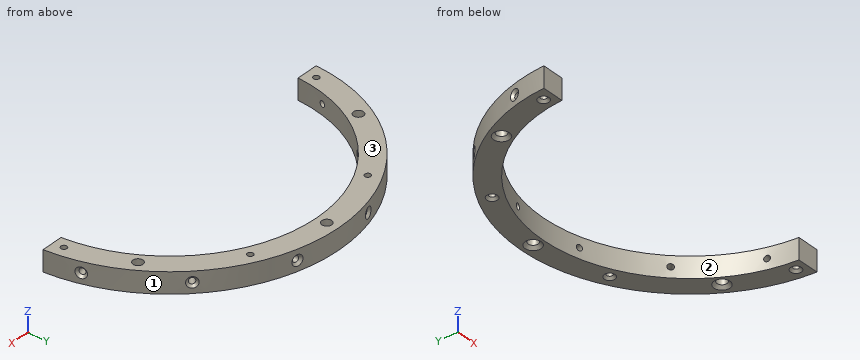
from build123d import *

# Parameters (mm, degrees)
BOSS_EXTRUDE1_DEPTH              = 3.96875
CIRPATTERN1_COUNT                = 6
CIRPATTERN1_ANGLE                = 150
F_4_40_TAPPED_HOLE3_D            = 2.2606
F_4_40_TAPPED_HOLE3_CSINK_D      = 4.1148
F_4_40_TAPPED_HOLE3_CSINK_ANGLE  = 90
CIRPATTERN2_COUNT                = 4
CIRPATTERN2_ANGLE                = 165
F_10_24_TAPPED_HOLE1_D           = 3.7973
F_10_24_TAPPED_HOLE1_CSINK_D     = 6.096
F_10_24_TAPPED_HOLE1_CSINK_ANGLE = 90
CIRPATTERN3_COUNT                = 3
CIRPATTERN3_ANGLE                = 120


with BuildPart() as part:
    # Sketch1 → Boss-Extrude1 (new body, symmetric)
    with BuildSketch(Plane.XY):
        with BuildLine():
            Line((-64.387964714, 3.8), (-55.87092267, 3.8))
            ThreePointArc((-55.87092267, 3.8), (0, 56), (55.87092267, 3.8))
            Line((55.87092267, 3.8), (64.387964714, 3.8))
            ThreePointArc((64.387964714, 3.8), (0, 64.5), (-64.387964714, 3.8))
        make_face()
    extrude(amount=BOSS_EXTRUDE1_DEPTH, both=True)

    # Sketch3 → #4-40 Tapped Hole2 (revolve, cut)
    with BuildSketch(Plane(origin=(62.302215796, 16.693828409, 0), x_dir=(-0.258819045, 0.965925826, 0), z_dir=(0, 0, 1))):
        Polygon((0, 0), (0, 9.549152758), (1.1303, 8.87), (1.1303, 0.9271), (2.0574, 0), align=None)
    f_4_40_tapped_hole2 = revolve(axis=Axis((68.435844793, 18.337329346, 0), (-0.965925826, -0.258819045, 0)), mode=Mode.SUBTRACT)

    # CirPattern1: #4-40 Tapped Hole2 ×6 about axis
    cirpattern1_axis = Axis((0, 0, 3.96875), (0, 0, 1))
    for i in range(1, CIRPATTERN1_COUNT):
        add(f_4_40_tapped_hole2.rotate(cirpattern1_axis, i * CIRPATTERN1_ANGLE / (CIRPATTERN1_COUNT - 1)), mode=Mode.SUBTRACT)

    # #4-40 Tapped Hole3 (through all)
    with Locations(Plane(origin=(0, 0, -3.96875), x_dir=(-1, 0, 0), z_dir=(0, 0, -1))):
        with Locations((-59.486691682, 7.831571533)):
            f_4_40_tapped_hole3 = CounterSinkHole(F_4_40_TAPPED_HOLE3_D / 2, F_4_40_TAPPED_HOLE3_CSINK_D / 2, counter_sink_angle=F_4_40_TAPPED_HOLE3_CSINK_ANGLE)

    # CirPattern2: #4-40 Tapped Hole3 ×4 about axis
    cirpattern2_axis = Axis((0, 0, 0), (0, 0, 1))
    for i in range(1, CIRPATTERN2_COUNT):
        add(f_4_40_tapped_hole3.rotate(cirpattern2_axis, i * CIRPATTERN2_ANGLE / (CIRPATTERN2_COUNT - 1)), mode=Mode.SUBTRACT)

    # #10-24 Tapped Hole1 (through all)
    with Locations(Plane(origin=(0, 0, -3.96875), x_dir=(-1, 0, 0), z_dir=(0, 0, -1))):
        with Locations((-51.961524227, 30)):
            f_10_24_tapped_hole1 = CounterSinkHole(F_10_24_TAPPED_HOLE1_D / 2, F_10_24_TAPPED_HOLE1_CSINK_D / 2, counter_sink_angle=F_10_24_TAPPED_HOLE1_CSINK_ANGLE)

    # CirPattern3: #10-24 Tapped Hole1 ×3 about axis
    cirpattern3_axis = Axis((0, 0, 0), (0, 0, 1))
    for i in range(1, CIRPATTERN3_COUNT):
        add(f_10_24_tapped_hole1.rotate(cirpattern3_axis, i * CIRPATTERN3_ANGLE / (CIRPATTERN3_COUNT - 1)), mode=Mode.SUBTRACT)


solid = part.part
CAD build for the part. Positions are in the model's coordinates, mm. Face numbers are marked on the shaded views. Give positions to 0.01 mm unless a question says otherwise; leave off trailing zeros. Order: outer loops, then holes, each group sorted by start corner. A loop starts at its lowest first (then second) coordinate and runs counter-clockwise, first axis right, second up. Notation, with made-up numbers: (68, 47) -> (121, 47) arc R8 cw to (121, 51) -> close; hole circle Ø9 at (39, 11). An arc over 180 degrees is marked (long way). Return JSON: item names as keys, results as strings.
Q1. Drill centre lines: line 1 (X direction, y = 30, z = -1); line 2 (X direction, y = 31.5, z = -3); line 3 (Y direction, x = 56.5, z = 1). Where is each one in solid material? Low to high.
Working result:
{"line 1": "-57.1 to -53.86, -50.06 to -47.29, 47.29 to 50.06, 53.86 to 57.1", "line 2": "-56.28 to -53.4, -50.52 to -46.3, 46.3 to 50.52, 53.4 to 56.28", "line 3": "3.8 to 14.59, 15.68 to 31.11"}
Q2. Saw through at A-A (y = 20). Write the cut outline in (x, z), then the cut area to 3 significant figures.
Working result:
{"outline": "(-61.32, -3.97) -> (-52.31, -3.97) -> (-52.31, 3.97) -> (-61.32, 3.97) -> close; (52.31, -3.97) -> (61.32, -3.97) -> (61.32, 3.97) -> (52.31, 3.97) -> close", "area": "143 mm²"}
Q3. Mould opens along X. For the marked faces 1, 2 and 3 say: pulls with the +X half, pulls with the -X half, needs draft (parallel to the pull), parting line crosses it, or undercut.
Working result:
{"face 1": "parting line crosses it", "face 2": "undercut", "face 3": "needs draft"}
Q4. Saw through at B-B (y = 30). Write the cut outline in (x, z), then the cut area to 3 significant figures.
Working result:
{"outline": "(-57.1, -3.97) -> (-55.01, -3.97) -> (-53.86, -2.82) -> (-53.86, 3.97) -> (-57.1, 3.97) -> close; (-50.06, -2.82) -> (-48.91, -3.97) -> (-47.29, -3.97) -> (-47.29, 3.97) -> (-50.06, 3.97) -> close; (47.29, -3.97) -> (48.91, -3.97) -> (50.06, -2.82) -> (50.06, 3.97) -> (47.29, 3.97) -> close; (53.86, -2.82) -> (55.01, -3.97) -> (57.1, -3.97) -> (57.1, 3.97) -> (53.86, 3.97) -> close", "area": "92.8 mm²"}
Q5. Flat gauge pins, fed straight in: pin 1 (2 mm diameter, centred on x = 31, z = 2.5, fed in from -Y); pin 2 (3 mm diameter, centred on x = -11.5, z = -2.5, fed in from -Y); pin 3 (3.5 mm diameter, centred on x = 0, y = 60, fed in from -Z); pin 4 (3 mm diameter, centred on x = 27.7, y = 53.22, fed in from +Z). Where does each tip first touch, or does it go through?
Working result:
{"pin 1": "y = 45.96", "pin 2": "y = 54.47", "pin 3": "through", "pin 4": "z = 3.97"}
